Part model, mm, in its own coordinate system. A direction names the side the tool comes from. Give positions to 0.01 mm unless a question says otherwise; leave off trailing zeros. Write each loop counter-clockwise with the first axis right and the second up, starting at its lowest first coordinate (ties: lowest second). Pieces come first, ordered by that corner, then holes.
from build123d import *

# Parameters (mm, degrees)
F2_R     = 1.1
F3_DEPTH = 7
F5_DEPTH = 6.5


with BuildPart() as f1:
    # F0 (on Front) → F1 (revolve)
    with BuildSketch(Plane.XZ):
        Polygon((18.140339697, 28.0600738525), (-32.159660303, 28.0600738525), (-32.159660303, 26.5600738525), (50.240339697, 26.5600738525), (50.240339697, 29.1100738525), (36.640339697, 29.1100738525), (36.640339697, 30.4600738525), (43.740339697, 30.4600738525), (43.740339697, 33.5600738525), (42.140339697, 33.5600738525), (42.140339697, 32.1600738525), (33.140339697, 32.1600738525), (33.140339697, 28.6600738525), (18.140339697, 28.6600738525), align=None)
    revolve(axis=Axis((9.040339697, 0, 26.5600738525), (-1, 0, 0)))

    # F2 (on face) → F3 (cut)
    with BuildSketch(Plane.YZ.offset(50.240339697)):
        with Locations((0, 26.5600738525)):
            Circle(F2_R)
    extrude(amount=-F3_DEPTH, mode=Mode.SUBTRACT)

    # F4 (on face) → F5 (join, through all)
    with BuildSketch(Plane.YZ.offset(50.240339697)):
        with BuildLine():
            Line((-1.23, 31.5938151088), (-1.23, 28.7938151088))
            ThreePointArc((-1.23, 28.7938151088), (0, 29.1100738525), (1.23, 28.7938151088))
            Line((1.23, 28.7938151088), (1.23, 31.5938151088))
            Line((1.23, 31.5938151088), (-1.23, 31.5938151088))
        make_face()
    extrude(amount=-F5_DEPTH)


solid = f1.part
1) Saw through at C-C (y = 4.75). Write the cut outline in (x, z), and give its area (3 significant figures).
Check result:
outline: (33.14, 23.59) - (42.14, 23.59) - (42.14, 21.42) - (43.74, 21.42) - (43.74, 31.7) - (42.14, 31.7) - (42.14, 29.53) - (33.14, 29.53) - close
area: 69.8 mm2
2) Flat gauge pins, fed straight in: P1, Ø5, axis at x = -3, z = 23.5, coming from the -Y side; P2, Ø3, axis at x = -16, z = 29, coming from the -Y side; P3, Ø3, axis at y = -2, z = 31.5, coming from the -X side; P4, Ø5, axis at x = -15, z = 32, coming from the +Y side. Where does each tip first touch, or does it go through?
Check result:
P1: stops at y = -1.39
P2: stops at y = -1.17
P3: stops at x = 33.14
P4: passes through
3) Saw through at B-B (x = 38). Write the cut outline in (y, z).
Check result:
outline: circle Ø11.2 at (0, 26.56); circle Ø5.1 at (0, 26.56); hole circle Ø7.8 at (0, 26.56)
4) Mould opens along Z. For faces 6 (the flat face through (47, 1.23, 30)), 7 (the flat face through (43.24, 0, 27)), 8 (the flat face through (47, 0, 31.594)) say: +Z half, -Z half, draft (parallel to the pull), parting line (faces both ways), or undercut.
Check result:
face 6: draft
face 7: undercut
face 8: +Z half
5) Saw through at D-D (x = -26.5). Write the cut outline in (y, z), and give its area (3 significant figures).
Check result:
outline: circle Ø3 at (0, 26.56)
area: 7.07 mm2
6) Drill centre lines: L1, parallel to Y at x = 41, z = 25.75; L2, parallel to X at y = 2.75, z = 31; L3, parallel to X at y = -0.25, z = 25. Where is each one in solid material? Low to high.
Check result:
L1: y = -5.54 to -3.81, -2.42 to 2.42, 3.81 to 5.54
L2: x = 33.14 to 43.74
L3: x = 18.14 to 50.24
7) 3-axis set-ups, long thin cutter, end or side, ignore diameter. For faces 1 (the flat face through (42.14, 5, 23)), 2 (the cylindrical face through (42.929, 2.103, 33.237)), 3 (the flat face through (-32.16, 0, 27)), 4 (the cylindrical face through (43.345, 0.112, 24.013)), 5 (the flat face through (47, -1.23, 30)): which of +Z, -Z, +X, -X, +Y, -Y reach the whole face in a straight line?
Check result:
face 1: -X
face 2: +X, -X
face 3: +Z, -Z, -X, +Y, -Y
face 4: none
face 5: +Z, +X, -Y
